```python
from build123d import *

# Parameters (mm, degrees)
SKETCH1_R           = 25.65
SKETCH1_R_2         = 19.65
SKETCH1_R_3         = 4
SKETCH1_R_4         = 0.95
BOSS_EXTRUDE1_DEPTH = 3.7
SKETCH2_R           = 25.65
SKETCH2_R_2         = 19.65
SKETCH2_R_3         = 4
SKETCH2_R_4         = 0.95
BOSS_EXTRUDE2_DEPTH = 50
SKETCH3_R           = 1.45
CUT_EXTRUDE1_DEPTH  = 15


with BuildPart() as part:
    # Sketch1 → Boss-Extrude1 (new body)
    # profile 1 of 2: a face of its own
    with BuildSketch(Plane(origin=(0, 0, 0), x_dir=(1, 0, 0), z_dir=(0, 1, 0))):
        with Locations(Location((0, 0, 0), (0, 0, 270))):
            Circle(SKETCH1_R)
        Circle(SKETCH1_R_2, mode=Mode.SUBTRACT)
    # profile 2 of 2: a face of its own
    with BuildSketch(Plane(origin=(0, 0, 0), x_dir=(1, 0, 0), z_dir=(0, 1, 0))):
        Circle(SKETCH1_R_2)
        with Locations(Location((0, 0, 0), (0, 0, 270))):
            Circle(SKETCH1_R_3, mode=Mode.SUBTRACT)
        with Locations(Location((16.6, 0, 0), (0, 0, 270))):
            Circle(SKETCH1_R_4, mode=Mode.SUBTRACT)
        with Locations(Location((0, -16.6, 0), (0, 0, 270))):
            Circle(SKETCH1_R_4, mode=Mode.SUBTRACT)
        with Locations(Location((-16.6, 0, 0), (0, 0, 270))):
            Circle(SKETCH1_R_4, mode=Mode.SUBTRACT)
        with Locations(Location((0, 16.6, 0), (0, 0, 270))):
            Circle(SKETCH1_R_4, mode=Mode.SUBTRACT)
    extrude(amount=BOSS_EXTRUDE1_DEPTH)

    # Sketch2 → Boss-Extrude2 (add)
    # profile 1 of 6: a face of its own
    with BuildSketch(Plane(origin=(0, 3.7, 0), x_dir=(1, 0, 0), z_dir=(0, 1, 0))):
        with Locations(Location((0, 0, 0), (0, 0, 270))):
            Circle(SKETCH2_R)
        with Locations(Location((0, 0, 0), (0, 0, 270))):
            Circle(SKETCH2_R_2, mode=Mode.SUBTRACT)
    # profile 2 of 6: a face of its own
    with BuildSketch(Plane(origin=(0, 3.7, 0), x_dir=(1, 0, 0), z_dir=(0, 1, 0))):
        with Locations(Location((0, 0, 0), (0, 0, 270))):
            Circle(SKETCH2_R_3)
    # profile 3 of 6: a face of its own
    with BuildSketch(Plane(origin=(0, 3.7, 0), x_dir=(1, 0, 0), z_dir=(0, 1, 0))):
        with Locations(Location((0, 16.6, 0), (0, 0, 270))):
            Circle(SKETCH2_R_4)
    # profile 4 of 6: a face of its own
    with BuildSketch(Plane(origin=(0, 3.7, 0), x_dir=(1, 0, 0), z_dir=(0, 1, 0))):
        with Locations(Location((-16.6, 0, 0), (0, 0, 270))):
            Circle(SKETCH2_R_4)
    # profile 5 of 6: a face of its own
    with BuildSketch(Plane(origin=(0, 3.7, 0), x_dir=(1, 0, 0), z_dir=(0, 1, 0))):
        with Locations(Location((0, -16.6, 0), (0, 0, 270))):
            Circle(SKETCH2_R_4)
    # profile 6 of 6: a face of its own
    with BuildSketch(Plane(origin=(0, 3.7, 0), x_dir=(1, 0, 0), z_dir=(0, 1, 0))):
        with Locations(Location((16.6, 0, 0), (0, 0, 270))):
            Circle(SKETCH2_R_4)
    extrude(amount=BOSS_EXTRUDE2_DEPTH)


with BuildPart() as boss_extrude2_kept_piece:
    # of the separate pieces the step leaves, the one the design keeps (boss_extrude2_pieces_kept)
    add(part.part.solids().sort_by_distance((0, 0, 25.65))[0])

    # Sketch3 → Cut-Extrude1 (cut)
    with BuildSketch(Plane(origin=(0, 53.7, 0), x_dir=(1, 0, 0), z_dir=(0, 1, 0))):
        with Locations(Location((22.65, 0, 0), (0, 0, 270))):
            Circle(SKETCH3_R)
        with Locations(Location((0, -22.65, 0), (0, 0, 270))):
            Circle(SKETCH3_R)
        with Locations(Location((-22.65, 0, 0), (0, 0, 270))):
            Circle(SKETCH3_R)
        with Locations(Location((0, 22.65, 0), (0, 0, 270))):
            Circle(SKETCH3_R)
    extrude(amount=-CUT_EXTRUDE1_DEPTH, mode=Mode.SUBTRACT)


solid = boss_extrude2_kept_piece.part
```
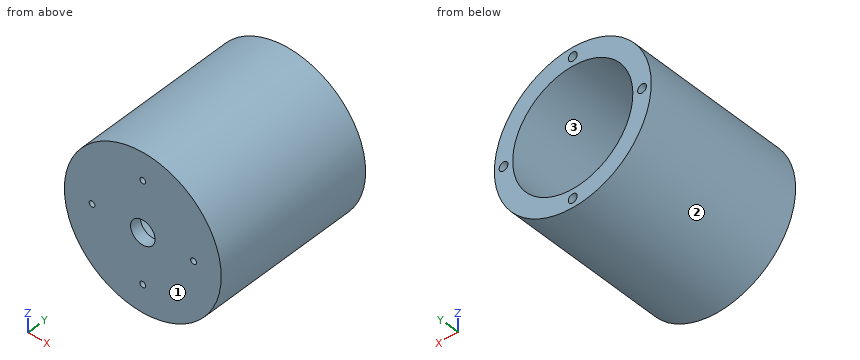
Geometry check sheet. Reference: the model listing, model coordinates, mm. Face numbers are marked on the shaded views. Coordinates: 2 decimals unless noted, no trailing zeros. Order: outer loops, then holes, each group sorted by start corner. A loop starts at its lowest first (then second) coordinate and runs counter-clockwise, first axis right, second up. Notation, with made-up numbers: (-32.75, -25) - (-15.75, -25) arc R37 ccw to (-15.75, 12) - close; hole circle Ø11 at (55, 63.25). An arc over 180 degrees is marked (long way). Answer in a Markdown table with one row per item. Add a question column.
1. Draft check along X on the marked faces 1, 2 and 3. Enter one of: +X half, -X half, draft (parallel to the pull), parting line (faces both ways), or undercut.
2. Section check B-B (y = 48.5). Enter the section's corners in (x, z), plus the area to 3 significant figures.
3. Section check A-A (z = 0). Enter the section's corners in (x, y), plus the area to 3 significant figures.
4. Section check D-D (x = 0). Enter the section's corners in (y, z), plus the area to 3 significant figures.
5. Gauge pin test, flat ends, axial feed: pin 1 Ø8 at (x, y) = (5.5, 39.5) entering from +Z; pin 2 Ø10 at (y, z) = (37, -11) entering from +X; pin 3 Ø5 at (x, y) = (18.5, 17) entering from +Z. Record the tip position at first contact, or that the pin passes through.
6. Material ranges on L1, parallel to X at y = 42, z = 0; L2, parallel to X at y = 1.05, z = 0; L3, parallel to Y at x = -23, z = -1, recorded low to high. Write a range as [from, to].
7. Section check C-C (x = -16.6). Enter the section's corners in (y, z).
Data:
| question | item | result |
|---|---|---|
| 1 | face 1 | draft |
| 1 | face 2 | parting line |
| 1 | face 3 | undercut |
| 2 | outline | circle Ø51.3 at (0, 0); hole circle Ø2.9 at (-22.65, 0); hole circle Ø39.3 at (0, 0); hole circle Ø2.9 at (0, -22.65); hole circle Ø2.9 at (0, 22.65); hole circle Ø2.9 at (22.65, 0) |
| 2 | area | 827 mm² |
| 3 | outline | (-25.65, 0) - (-17.55, 0) - (-17.55, 3.7) - (-19.65, 3.7) - (-19.65, 53.7) - (-21.2, 53.7) - (-21.2, 38.7) - (-24.1, 38.7) - (-24.1, 53.7) - (-25.65, 53.7) - close; (-15.65, 0) - (-4, 0) - (-4, 3.7) - (-15.65, 3.7) - close; (4, 0) - (15.65, 0) - (15.65, 3.7) - (4, 3.7) - close; (17.55, 0) - (25.65, 0) - (25.65, 53.7) - (24.1, 53.7) - (24.1, 38.7) - (21.2, 38.7) - (21.2, 53.7) - (19.65, 53.7) - (19.65, 3.7) - (17.55, 3.7) - close |
| 3 | area | 659 mm² |
| 4 | outline | (0, -25.65) - (53.7, -25.65) - (53.7, -24.1) - (38.7, -24.1) - (38.7, -21.2) - (53.7, -21.2) - (53.7, -19.65) - (3.7, -19.65) - (3.7, -17.55) - (0, -17.55) - close; (0, -15.65) - (3.7, -15.65) - (3.7, -4) - (0, -4) - close; (0, 4) - (3.7, 4) - (3.7, 15.65) - (0, 15.65) - close; (0, 17.55) - (3.7, 17.55) - (3.7, 19.65) - (53.7, 19.65) - (53.7, 21.2) - (38.7, 21.2) - (38.7, 24.1) - (53.7, 24.1) - (53.7, 25.65) - (0, 25.65) - close |
| 4 | area | 659 mm² |
| 5 | pin 1 | stops at z = 25.61 |
| 5 | pin 2 | stops at x = 24.94 |
| 5 | pin 3 | stops at z = 20.05 |
| 6 | L1 | x = [-25.65, -24.1], [-21.2, -19.65], [19.65, 21.2], [24.1, 25.65] |
| 6 | L2 | x = [-25.65, -17.55], [-15.65, -4], [4, 15.65], [17.55, 25.65] |
| 6 | L3 | y = [0, 38.7] |
| 7 | outline | (0, -19.55) - (53.7, -19.55) - (53.7, -10.51) - (3.7, -10.51) - (3.7, -0.95) - (0, -0.95) - close; (0, 0.95) - (3.7, 0.95) - (3.7, 10.51) - (53.7, 10.51) - (53.7, 19.55) - (0, 19.55) - close |
